Input: part model. Units: mm. Frame: model coordinates. A direction names the side the tool comes from. Coordinates: 2 decimals unless noted, no trailing zeros. Write each loop counter-clockwise with the first axis right and the second up, starting at its lowest first coordinate (ties: lowest second). Pieces come first, ordered by that corner, then holes.
Autodesk Inventor part; units mm, degrees
ref_plane "РабПлоскость8" through (0, 470, 32) normal (-0.5031, 0.3593, -0.786) x (0.8423, 0, -0.5391)
ref_plane "РабПлоскость9" through (290, 470, 32) normal (-0.5031, -0.3593, 0.786) x (-0.8423, 0, -0.5391)
ref_plane "РабПлоскость10" through (0, 0, 32) normal (0.4634, 0.1738, 0.8689) x (0.8824, 0, -0.4706)
sketch "Эскиз1" plane through (0, 0, 0) normal (0, 0, 1) x (1, 0, 0)
  line L0 (0, 0) -> (290, 0)
  line L1 (290, 0) -> (290, 470)
  line L2 (290, 470) -> (0, 470)
  line L3 (0, 470) -> (0, 0)
  line L4 (145, 470) -> (145, 0) construction
  circle A0 centre (145, 180) radius 133
  circle A1 centre (145, 180) radius 115
  circle A2 centre (80, 390) radius 47
  circle A3 centre (80, 390) radius 30
  line L5 (138.0736, 432.9264) -> (229.9264, 432.9264)
  line L6 (236.9264, 425.9264) -> (236.9264, 334.0736)
  line L7 (229.9264, 327.0736) -> (138.0736, 327.0736)
  line L8 (131.0736, 334.0736) -> (131.0736, 425.9264)
  line L9 (131.0736, 432.9264) -> (236.9264, 327.0736) construction
  line L10 (236.9264, 432.9264) -> (131.0736, 327.0736) construction
  circle A4 centre (184, 380) radius 47
  circle A5 centre (184, 380) radius 58 construction
  line L11 (0, 160) -> (60, 0)
  line L12 (290, 160) -> (230, 0)
  line L13 (50, 470) -> (0, 400)
  line L14 (240, 470) -> (290, 400)
  line L15 (290, 320) -> (0, 320) construction
  arc A6 (236.9264, 428.9264) -> (232.9264, 432.9264) centre (232.9264, 428.9264) ccw
  arc A7 (236.9264, 425.9264) -> (229.9264, 432.9264) centre (229.9264, 425.9264) ccw
  arc A8 (138.0736, 432.9264) -> (131.0736, 425.9264) centre (138.0736, 425.9264) ccw
  arc A9 (131.0736, 334.0736) -> (138.0736, 327.0736) centre (138.0736, 334.0736) ccw
  arc A10 (229.9264, 327.0736) -> (236.9264, 334.0736) centre (229.9264, 334.0736) ccw
  line L16 (0, 320) -> (290, 320)
  dimension "d0" = 290
  dimension "d1" = 470
  dimension "d3" = 266
  dimension "d4" = 230
  dimension "d5" = 94
  dimension "d6" = 60
  dimension "d9" = 94
  dimension "d11" = 380
  dimension "d12" = 390
  dimension "d13" = 180
  dimension "d16" = 160
  dimension "d17" = 60
  dimension "d20" = 80
  dimension "d21" = 50
  dimension "d38" = 70
  dimension "d39" = 320
  dimension "d51" = 106
extrude "Выдавливание1" add sketch "Эскиз1" along normal blind 42 contours L3 L11 L0 | L11 L3 L16 L1 L12 L0 | L12 L1 L0 | L3 L13 L2 L14 L1 L16 | L3 L2 L13 | L14 L2 L1 | A0 | A2 | L5 A7 L6 A10 L7 A9 L8 A8
sketch "Эскиз3" plane through (0, 470, 0) normal (0, 1, 0) x (1, 0, 0)
  line L0 (290, 0) -> (290, -42)
  line L1 (0, 0) -> (0, -42)
  point P0 (290, -32)
  point P1 (0, -32)
  dimension "d24" = 10
  dimension "d25" = 10
sketch "Эскиз4" plane through (0, 0, 0) normal (0, -1, 0) x (1, 0, 0)
  line L0 (0, 0) -> (0, 42)
  line L1 (290, 0) -> (290, 42)
  point P0 (0, 32)
  point P1 (290, 32)
chamfer "Фаска2" distance 10 distance2 30 1 edges at (30, 180, 42) measured on face at (145, 21.6667, 42)
chamfer "Фаска3" distance 10 angle 45 1 edges at (137, 380, 42)
ref_plane "РабПлоскость8" through (0, 470, 32) normal (-0.5031, 0.3593, -0.786) x (0.8423, 0, -0.5391)
split "Разделение8" plane through (0, 470, 32) removes the side toward (-0.5031, 0.3593, -0.786)
ref_plane "РабПлоскость9" through (290, 470, 32) normal (-0.5031, -0.3593, 0.786) x (-0.8423, 0, -0.5391)
split "Разделение9" plane through (290, 470, 32) removes the side toward (0.5031, 0.3593, -0.786)
ref_plane "РабПлоскость10" through (0, 0, 32) normal (0.4634, 0.1738, 0.8689) x (0.8824, 0, -0.4706)
split "Разделение10" plane through (0, 0, 32) removes the side toward (-0.4634, -0.1738, -0.8689)
ref_plane "РабПлоскость11" through (290, 0, 32) normal (-0.4634, 0.1738, 0.8689) x (0, 0.9806, -0.1961)
split "Разделение11" plane through (290, 0, 32) removes the side toward (0.4634, -0.1738, -0.8689)
chamfer "Фаска5" distance 4 angle 45 4 edges at (290, 280, 0) (145, 470, 0) (0, 280, 0) (145, 0, 0)
extrude "Выдавливание2" cut sketch "Эскиз1" along normal blind 4 contours A0 | A1
extrude "Выдавливание3" cut sketch "Эскиз1" along normal blind 4 contours A2
extrude "Выдавливание4" cut sketch "Эскиз1" along normal blind 2 contours L5 A7 L6 A10 L7 A9 L8 A8
properties part number "Front" material "Пластик АБС"
Item 1: Section query C-C, the plane y = 380. Return loops of the section in (x, z), then the cut area to 3 significant figures.
Item 2: Access query for faces 1 (the face through (79, 291, 42)), 2 (the face through (183, 428, 2)). Directions: +Z, -Z, +X, -X, +Y, -Y. A direction counts if a zero-diameter tool reaches every point of the face in a straight line with its end or side. Return the directions, or none.
Item 3: Material intervals for line 1 (Y direction, x = 187, z = 18); line 2 (Y direction, x = 194.5, z = 14.5); line 3 (X direction, y = 159, z = 38), sorted ascending.
Item 4: Pin query (flat end, axial travel): pin 1 Ø2 at (y, z) = (364.5, 1) entering from -X; pin 2 Ø1.6 at (y, z) = (399, 1) entering from +X; pin 3 Ø1.6 at (x, z) = (201.5, 0.5) entering from +Y. Return the tip coordinate at first contact, or that it passes through.
Item 5: Section query D-D, the plane x = 83.5. State how many separate pieces and enclosed holes the cut face has, then the cut area to 3 significant figures.
Item 6: Section query A-A, the plane y = 180. Return loops of the section in (x, z).
Item 7: Section query B-B, the plane z = 21.5. Return loops of the section in (x, y).
Item 8: Pull-direction query (X, two-part tool) for faces 3 (the face through (290, 232, 23)), 4 (the face through (73.88, 343.4, 1.97)), 5 (the face through (0, 238, 23)); classes: released by +X, released by -X, zero draft, split by the parting line, or undercut.
The answers:
1. outline: (0, 4) - (4, 0) - (34.08, 0) - (34.08, 4) - (51.72, 4) - (51.72, 42) - (0, 42) - close; (108.28, 4) - (125.92, 4) - (125.92, 0) - (131.07, 0) - (131.07, 2) - (137, 2) - (137, 32) - (127, 42) - (108.28, 42) - close; (231, 2) - (236.93, 2) - (236.93, 0) - (286, 0) - (290, 4) - (290, 42) - (241, 42) - (231, 32) - close
1. area: 5,580 mm2
2. face 1: +Z, +X, -X, +Y, -Y
2. face 2: -Z
3. line 1: y = 0 to 70.8, 289.2 to 333.1, 426.9 to 470
3. line 2: y = 0 to 75.28, 284.72 to 334.19, 425.81 to 470
3. line 3: x = 0 to 23.13, 266.87 to 290
4. pin 1: stops at x = 2
4. pin 2: stops at x = 287.8
4. pin 3: stops at y = 467.3
5. separate pieces: 3
5. enclosed holes: 0
5. area: 8,400 mm2
6. outline: (0, 4) - (4, 0) - (12, 0) - (12, 4) - (30, 4) - (30, 12) - (20, 42) - (0, 42) - close; (260, 4) - (278, 4) - (278, 0) - (286, 0) - (290, 4) - (290, 42) - (270, 42) - (260, 12) - close
7. outline: (0, 52.49) - (19.69, 0) - (270.31, 0) - (290, 52.49) - (290, 447.03) - (273.6, 470) - (16.4, 470) - (0, 447.03) - close; hole circle Ø236.33 at (145, 180); hole circle Ø60 at (80, 390); hole circle Ø94 at (184, 380)
8. face 3: released by +X
8. face 4: undercut
8. face 5: released by -X
